Read the model definition and answer for the solid it produces. Units are mm, in the model's axes. Face numbers are marked on the shaded views. A direction names the side the tool comes from. Give positions to 0.01 mm unless a question says otherwise; leave off trailing zeros. Order: outer loops, then holes, each group sorted by start corner. A loop starts at its lowest first (then second) coordinate and runs counter-clockwise, first axis right, second up. Notation, with made-up numbers: M -10,81.25 L 12,81.25 A16 cw 12,109.25 Z; hole C 7.5,45 d3. An arc over 180 degrees is marked long. Write item = value, one per line. Start each with the question number.
from build123d import *

# Parameters (mm, degrees)
SKETCH3_R           = 2
BOSS_EXTRUDE1_DEPTH = 3
SKETCH6_R           = 5
BOSS_EXTRUDE2_DEPTH = 37.5


with BuildPart() as part:
    # Sketch3 → Boss-Extrude1 (new, symmetric)
    with BuildSketch(Plane(origin=(0, 0, 0), x_dir=(1, 0, 0), z_dir=(0, 1, 0))):
        with BuildLine():
            Line((8.5, -6), (-8.5, -6))
            Line((-8.5, -6), (-8.5, 6))
            Line((-8.5, 6), (8.5, 6))
            ThreePointArc((8.5, 6), (14.5, 0), (8.5, -6))
        make_face()
        with Locations(Location((7, 0, 0), (0, 0, 270))):
            Circle(SKETCH3_R, mode=Mode.SUBTRACT)
    extrude(amount=BOSS_EXTRUDE1_DEPTH, both=True)

    # Sketch6 → Boss-Extrude2 (add, symmetric)
    with BuildSketch(Plane.XY):
        with Locations((-8.5, 0)):
            Circle(SKETCH6_R)
    extrude(amount=BOSS_EXTRUDE2_DEPTH, both=True)


solid = part.part
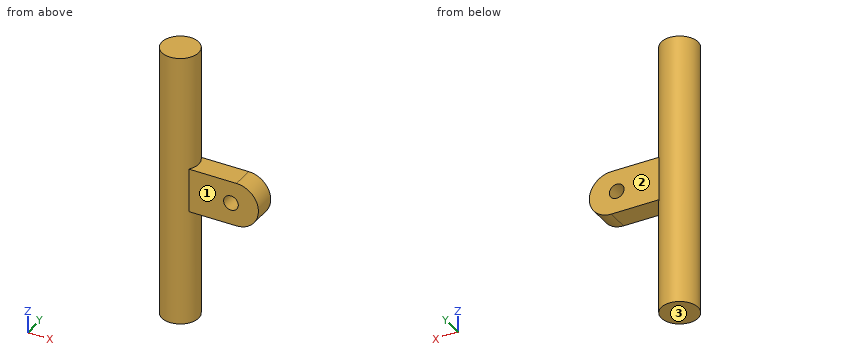
1) Find section A-A on y = 0. Determine the outline of the cut face in (x, z).
2) For the marked faces 1, 2 and 3, determine the directions among +Z, -Z, +X, -X, +Y, -Y from which every point of the face is accessible in a straight line to the end or side of a thin tool.
3) Find the intervals of material crossed by probe 1 along X at (y, z) = (0.4, 0); probe 2 along X at (y, z) = (0.85, 0); probe 3 along Z at (x, y) = (0.75, 2.25), in increasing order. Write a range as [from, to].
4) Find section C-C on x = 7. Determine the outline of the cut face in (y, z), plus the area to 3 significant figures.
5) Find section D-D on z = 32. Determine the outline of the cut face in (x, y).
6) Find section B-B on z = 0. Determine the outline of the cut face in (x, y), plus the area to 3 significant figures.
7) Each of these flat-tipped pins is pushed along its axis until it touches: P1, Ø5, axis at x = 2.5, y = 1, coming from the -Z side; P2, Ø6, axis at x = 0.5, z = 11, coming from the -Y side; P3, Ø9.5, axis at x = 4, z = 2, coming from the +Y side; P4, Ø2, axis at y = -3.5, z = -10.5, coming from the +X side. Where does it stop, or does it pass through?
Numbers:
q1.outline = M -13.5,-37.5 L -3.5,-37.5 L -3.5,-6 L 8.5,-6 A6 ccw 8.5,6 L -3.5,6 L -3.5,37.5 L -13.5,37.5 Z; hole C 7,0 d4
q2.face_1 = +Z, -Z, +X, -Y
q2.face_2 = +Z, -Z, +X, +Y
q2.face_3 = -Z, +X, -X, +Y, -Y
q3.probe_1 = [-13.48, 5], [9, 14.5]
q3.probe_2 = [-13.43, 5], [9, 14.5]
q3.probe_3 = [-6, 6]
q4.outline = M -3,-6 L 3,-6 L 3,-2 L -3,-2 Z; M -3,2 L 3,2 L 3,6 L -3,6 Z
q4.area = 48.0 mm2
q5.outline = C -8.5,0 d10
q6.outline = M -4.5,-3 L 5,-3 L 5,3 L -4.5,3 A5 ccw long Z; M 9,-3 L 14.5,-3 L 14.5,3 L 9,3 Z
q6.area = 164 mm2
q7.P1 = -6
q7.P2 = through
q7.P3 = 3
q7.P4 = -4.17
